from build123d import *

# Parameters (mm, degrees)
F1_DEPTH = 3


with BuildPart() as f1:
    # F0 (on Top) → F1 (new body)
    with BuildSketch(Plane.XY):
        with BuildLine():
            Line((25, 3.365576), (0, 3.365576))
            Line((0, 3.365576), (-25, 3.365576))
            ThreePointArc((-25, 3.365576), (-22.87868, 2.486897), (-22, 0.365576))
            ThreePointArc((-22, 0.365576), (-22.87868, -1.755744), (-25, -2.634424))
            Line((-25, -2.634424), (0, -2.634424))
            Line((0, -2.634424), (25, -2.634424))
            ThreePointArc((25, -2.634424), (28, 0.365576), (25, 3.365576))
        make_face()
        with BuildLine():
            ThreePointArc((-18.5, -1.134424), (-20, 0.365576), (-18.5, 1.865576))
            Line((-18.5, 1.865576), (25, 1.865576))
            ThreePointArc((25, 1.865576), (26.06066, 1.426237), (26.5, 0.365576))
            ThreePointArc((26.5, 0.365576), (26.06066, -0.695084), (25, -1.134424))
            Line((25, -1.134424), (-18.5, -1.134424))
        make_face(mode=Mode.SUBTRACT)
        with BuildLine():
            ThreePointArc((-22, 0.365576), (-22.87868, 2.486897), (-25, 3.365576))
            ThreePointArc((-25, 3.365576), (-28, 0.365576), (-25, -2.634424))
            ThreePointArc((-25, -2.634424), (-22.87868, -1.755744), (-22, 0.365576))
        make_face()
        with BuildLine():
            ThreePointArc((-23.5, 0.365576), (-23.93934, -0.695084), (-25, -1.134424))
            ThreePointArc((-25, -1.134424), (-26.06066, 1.426237), (-23.5, 0.365576))
        make_face(mode=Mode.SUBTRACT)
    extrude(amount=F1_DEPTH)


solid = f1.part
Input: part model. Units: mm. Frame: model coordinates. A direction names the side the tool comes from. Round coordinates to 2 decimals unless told otherwise and drop trailing zeros. Write each loop counter-clockwise with the first axis right and the second up, starting at its lowest first coordinate (ties: lowest second). Pieces come first, ordered by that corner, then holes.
1) Reachability of faces 1 (the cylindrical face through (-20, 0.3, 1.5)), 2 (the flat face through (-0.4, 2.4, 0)) from +Z, -Z, +X, -X, +Y, -Y: full face, straight path, thin tool, end or side. Return the list, or none.
2) Ray query, L1, parallel to X at y = 0.25, z = 1.05; L2, parallel to Y at x = -4, z = 0.8; L3, parallel to X at y = 1, z = 1.1. Return the intervals inside material, ascending.
3) Cut plane B-B (z = 1.3). Return the cut outline in (x, y).
4) Cut plane A-A (x = 22). Return the cut outline in (y, z), then the cut area to 3 significant figures.
Geometry says:
1. face 1: +Z, -Z
1. face 2: -Z, +X, -X, +Y, -Y
2. L1: x = -28 to -26.5, -23.5 to -20, 26.5 to 28
2. L2: y = -2.63 to -1.13, 1.87 to 3.37
2. L3: x = -27.93 to -26.36, -23.64 to -19.86, 26.36 to 27.93
3. outline: (-25, -2.63) - (25, -2.63) arc R3 ccw to (25, 3.37) - (-25, 3.37) arc R3 ccw to start; hole circle Ø3 at (-25, 0.37); hole (-18.5, -1.13) - (25, -1.13) arc R1.5 ccw to (26.5, 0.37) arc R1.5 ccw to (25, 1.87) - (-18.5, 1.87) arc R1.5 ccw to start
4. outline: (-2.63, 0) - (-1.13, 0) - (-1.13, 3) - (-2.63, 3) - close; (1.87, 0) - (3.37, 0) - (3.37, 3) - (1.87, 3) - close
4. area: 9.00 mm2
